The listing builds one solid part. Answer for the finished solid, in the listing's coordinates (mm). Round coordinates to 2 decimals unless told otherwise and drop trailing zeros. Loops run counter-clockwise (first coordinate to the right, second up) from the corner with the lowest first, then second, coordinate; pieces in that order, holes last. Notation, with made-up numbers: M 37,-32.5 L 87,-32.5 A26 ccw 87,5.5 Z; hole C -24,73 d7. An arc over 180 degrees is marked long. Answer as a JSON object with one key per item and string values.
```python
from build123d import *

# Parameters (mm, degrees)
BOSS_EXTRUDE1_DEPTH = 2
SKETCH2_R           = 1
BOSS_EXTRUDE2_DEPTH = 3.8
SKETCH3_W           = 26
SKETCH3_H           = 30
BOSS_EXTRUDE3_DEPTH = 16
SKETCH4_W           = 24
SKETCH4_H           = 28
CUT_EXTRUDE1_DEPTH  = 26
SKETCH5_W           = 28
SKETCH5_H           = 14
CUT_EXTRUDE2_DEPTH  = 1
SKETCH6_W           = 28
SKETCH6_H           = 1
BOSS_EXTRUDE4_DEPTH = 25


with BuildPart() as part:
    # Sketch1 → Boss-Extrude1 (new body)
    with BuildSketch(Plane(origin=(0, 0, 0), x_dir=(1, 0, 0), z_dir=(0, 1, 0))):
        Polygon((0, 0), (66, 0), (66, -4), (71, -4), (71, -107), (60.8, -107), (60.8, -115), (60.8, -124), (5.2, -124), (5.2, -115), (5.2, -107), (-5, -107), (-5, -4), (0, -4), align=None)
    extrude(amount=BOSS_EXTRUDE1_DEPTH)

    # Sketch2 → Boss-Extrude2 (add)
    with BuildSketch(Plane(origin=(0, 2, 0), x_dir=(1, 0, 0), z_dir=(0, 1, 0))):
        with Locations(Location((10, -120, 0), (0, 0, 90))):
            Circle(SKETCH2_R)
        with Locations(Location((56, -120, 0), (0, 0, 90))):
            Circle(SKETCH2_R)
        with Locations(Location((2.5, -1.5, 0), (0, 0, 90))):
            Circle(SKETCH2_R)
        with Locations(Location((63.5, -1.5, 0), (0, 0, 90))):
            Circle(SKETCH2_R)
    extrude(amount=BOSS_EXTRUDE2_DEPTH)

    # Sketch3 → Boss-Extrude3 (add)
    with BuildSketch(Plane(origin=(0, 0, 0), x_dir=(-1, 0, 0), z_dir=(0, -1, 0))):
        with Locations((-44, -25)):
            Rectangle(SKETCH3_W, SKETCH3_H)
    extrude(amount=-BOSS_EXTRUDE3_DEPTH)

    # Sketch4 → Cut-Extrude1 (cut)
    with BuildSketch(Plane(origin=(0, 16, 0), x_dir=(1, 0, 0), z_dir=(0, 1, 0))):
        with Locations((44, -25)):
            Rectangle(SKETCH4_W, SKETCH4_H)
    extrude(amount=-CUT_EXTRUDE1_DEPTH, mode=Mode.SUBTRACT)

    # Sketch5 → Cut-Extrude2 (cut)
    with BuildSketch(Plane(origin=(32, 0, 0), x_dir=(0, 0, -1), z_dir=(1, 0, 0))):
        with Locations((-25, 9)):
            Rectangle(SKETCH5_W, SKETCH5_H)
    extrude(amount=-CUT_EXTRUDE2_DEPTH, mode=Mode.SUBTRACT)

    # Sketch6 → Boss-Extrude4 (add)
    with BuildSketch(Plane.ZY.offset(-56)):
        with Locations((25, 15.5)):
            Rectangle(SKETCH6_W, SKETCH6_H)
    extrude(amount=BOSS_EXTRUDE4_DEPTH)


solid = part.part
```
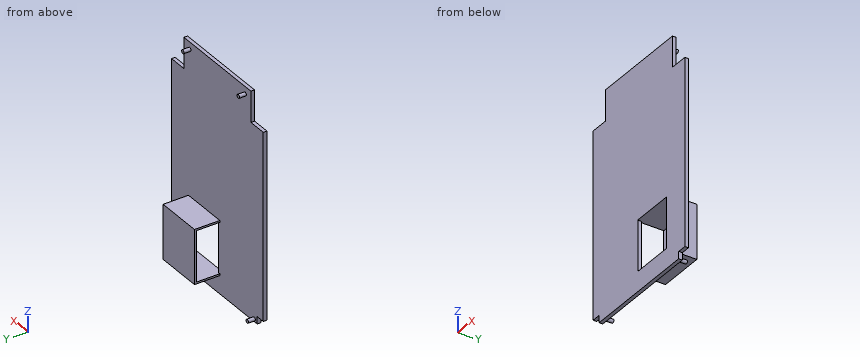
Item 1: The part is cut by section C-C (z = 110.5). Give the vertices of the cut face in (x, y).
Values follow:
{"outline": "M 5.2,0 L 60.8,0 L 60.8,2 L 5.2,2 Z"}
Item 2: Flat-ended cylindrical pins translate along their axes: P1, Ø1, axis at x = 63.5, z = 1, coming from the +Y side; P2, Ø6, axis at x = 27.5, z = 43.5, coming from the +Y side; P3, Ø2, axis at y = 7.5, z = 40.5, coming from the +X side. Find the tip coordinate at first contact, or state that the pin passes through.
Values follow:
{"P1": "y = 5.8", "P2": "y = 2", "P3": "x = 57"}
Item 3: The part is cut by section B-B (y = 13.5). Give the vertices of the cut face in (x, z), then the cut area to 3 significant figures.
Values follow:
{"outline": "M 31,10 L 57,10 L 57,40 L 31,40 L 31,39 L 56,39 L 56,11 L 31,11 Z", "area": "80.0 mm^2"}
Item 4: Straight lines are drawn through the part: line 1 (Z direction, x = 40, y = 8.25); line 2 (Y direction, x = 39.5, z = 100); line 3 (X direction, y = 3.5, z = 10.5). For each, find the intervals that lie inside material, in ascending order.
Values follow:
{"line 1": "10 to 11, 39 to 40", "line 2": "0 to 2", "line 3": "31 to 57"}
Item 5: The part is cut by section D-D (x = 14). Give the vertices of the cut face in (y, z), then the cut area to 3 significant figures.
Values follow:
{"outline": "M 0,0 L 2,0 L 2,124 L 0,124 Z", "area": "248 mm^2"}
Item 6: The part is cut by section A-A (z = 33.5). Give the vertices of the cut face in (x, y).
Values follow:
{"outline": "M -5,0 L 32,0 L 32,2 L -5,2 Z; M 31,15 L 56,15 L 56,0 L 71,0 L 71,2 L 57,2 L 57,16 L 31,16 Z"}
